Work out the finished part from the listing and answer in its coordinate system (mm). A direction names the side the tool comes from. Round coordinates to 2 decimals unless told otherwise and drop trailing zeros. Loops run counter-clockwise (first coordinate to the right, second up) from the corner with the lowest first, then second, coordinate; pieces in that order, holes last. Notation, with made-up numbers: M 52.5,76.5 L 68.5,76.5 A18 ccw 68.5,81.5 Z; hole C 66.25,88 d7. An arc over 180 degrees is marked long. One line per item, written item: value.
```python
from build123d import *

# Parameters (mm, degrees)
SKETCH1_R           = 12.630912
BOSS_EXTRUDE1_DEPTH = 71.882
SHELL1_T            = -0.6985
CUT_EXTRUDE1_DEPTH  = 71.882


with BuildPart() as part:
    # Sketch1 → Boss-Extrude1 (new body)
    with BuildSketch(Plane.XY):
        with Locations((-89.675021381, 9.53355709)):
            Circle(SKETCH1_R)
    extrude(amount=BOSS_EXTRUDE1_DEPTH)

    # Shell1
    shell1_openings = [part.faces().sort_by_distance(p)[0] for p in [
        (-89.675021381, 9.53355709, 71.882),
        (-89.675021381, 9.53355709, 0),
    ]]
    offset(amount=SHELL1_T, openings=shell1_openings, kind=Kind.INTERSECTION)

    # Sketch4 → Cut-Extrude1 (cut)
    with BuildSketch(Plane(origin=(-89.662, 0, 0), x_dir=(0, 0, -1), z_dir=(1, 0, 0))):
        with BuildLine():
            Line((-58.1025, 12.59425709), (-46.1391, 12.59425709))
            ThreePointArc((-46.1391, 12.59425709), (-43.0784, 9.53355709), (-46.1391, 6.47285709))
            Line((-46.1391, 6.47285709), (-58.1025, 6.47285709))
            ThreePointArc((-58.1025, 6.47285709), (-61.1632, 9.53355709), (-58.1025, 12.59425709))
        make_face()
    extrude(amount=CUT_EXTRUDE1_DEPTH, mode=Mode.SUBTRACT)


solid = part.part
```
1) Find section C-C (z = 50.5). Give the vertices of the cut face in (x, y), then the cut area to 3 significant figures.
Check values:
outline: M -78.14,6.47 A11.93 cw long -78.14,12.59 L -77.42,12.59 A12.63 ccw long -77.42,6.47 Z
area: 49.6 mm2
2) For faces 4 (the face through (-80, 17, 0)), 5 (the face through (-77.48, 9.6, 43.08)), determine the directions among +Z, -Z, +X, -X, +Y, -Y from which every point of the face is accessible in a straight line to the end or side of a thin tool.
Check values:
face 4: -Z, +X, -X, +Y, -Y
face 5: +X
3) The mould has two halves that part along X. Classify faces 1 (the face through (-102.294, 10.089, 35.438)), 2 (the face through (-80, 17, 71.882)), 3 (the face through (-92.262, -2.115, 35.438)): +X half, -X half, draft (parallel to the pull), parting line (faces both ways), or undercut.
Check values:
face 1: parting line
face 2: draft
face 3: undercut
4) Find section D-D (z = 16.5). Give the vertices of the cut face in (x, y), then the cut area to 3 significant figures.
Check values:
outline: C -89.68,9.53 d25.26; hole C -89.68,9.53 d23.86
area: 53.9 mm2
5) Each of these flat-tipped pins is pushed along its axis until it touches: pin 1 (8 mm diameter, centred on y = 0, z = 15, fed in from +X); pin 2 (12 mm diameter, centred on y = 11, z = 58.5, fed in from +X); pin 3 (4 mm diameter, centred on y = 5, z = 28, fed in from +X); pin 4 (5 mm diameter, centred on x = -93, y = 18, fed in from +Z). Where does it stop, or does it pass through?
Check values:
pin 1: x = -78.32
pin 2: x = -77.04
pin 3: x = -77.3
pin 4: through
6) Find section A-A (y = 18.5). Give the vertices of the cut face in (x, z).
Check values:
outline: M -98.57,0 L -97.55,0 L -97.55,71.88 L -98.57,71.88 Z; M -81.8,0 L -80.78,0 L -80.78,71.88 L -81.8,71.88 Z
7) Find the intervals of material crossed by probe 1 along X at (y, z) = (10, 42); probe 2 along X at (y, z) = (2.5, 23); probe 3 along Y at (x, z) = (-98, 33), in increasing order. Write a range as from..to.
Check values:
probe 1: -102.3..-101.6, -77.75..-77.05
probe 2: -100.17..-99.31, -80.04..-79.18
probe 3: 0.03..0.99, 18.08..19.03
8) Find section B-B (x = -93.5). Give the vertices of the cut face in (y, z).
Check values:
outline: M -2.5,0 L -1.77,0 L -1.77,71.88 L -2.5,71.88 Z; M 20.84,0 L 21.57,0 L 21.57,71.88 L 20.84,71.88 Z
